from build123d import *

# Parameters (mm, degrees)
F2_W        = 15
F2_H        = 19.25
F2_R        = 2.75
F3_DEPTH    = 40
F5_DEPTH    = 22.251
F6_W        = 6.75
F6_H        = 19.25
F6_W_2      = 20.5
F7_DEPTH    = 30.001
F8_T1_DEPTH = 15
F8_T3_DEPTH = 28
F8_T5_DEPTH = 28
F8_T7_DEPTH = 28
F10_R       = 2


# Not quite as in the source:
# - a fillet or chamfer that OpenCascade refuses, or shapes differently, is made with other operations: its cross-section is extruded or revolved along the edge and cut away or added
# - a feature of the source that left no trace in its solid (it failed there, or was rolled back) is left out


with BuildPart() as f3:
    # F2 (on Front) → F3 (new body)
    with BuildSketch(Plane.XZ):
        Polygon((-47, -12.4571), (-32, -12.4571), (-17, -12.4571), (-17, -9.4571), (-47, -9.4571), align=None)
        with Locations((-39.5, -22.0821)):
            Rectangle(F2_W, F2_H)
        with Locations((-39.5, -23.9571)):
            Circle(F2_R, mode=Mode.SUBTRACT)
    extrude(amount=F3_DEPTH)

    # F4 (on face) → F5 (cut, through all)
    with BuildSketch(Plane.XY.offset(-9.4571)):
        with BuildLine():
            Line((-24, -11.5), (-24, -6.5))
            ThreePointArc((-24, -6.5), (-26, -4.5), (-28, -6.5))
            Line((-28, -6.5), (-28, -11.5))
            ThreePointArc((-28, -11.5), (-26, -13.5), (-24, -11.5))
        make_face()
        with BuildLine():
            Line((-32, -22.5), (-32, -17.5))
            ThreePointArc((-32, -17.5), (-34, -15.5), (-36, -17.5))
            Line((-36, -17.5), (-36, -22.5))
            ThreePointArc((-36, -22.5), (-34, -24.5), (-32, -22.5))
        make_face()
        with BuildLine():
            ThreePointArc((-28, -33.5), (-26, -35.5), (-24, -33.5))
            Line((-24, -33.5), (-24, -28.5))
            ThreePointArc((-24, -28.5), (-26, -26.5), (-28, -28.5))
            Line((-28, -28.5), (-28, -33.5))
        make_face()
    extrude(amount=-F5_DEPTH, mode=Mode.SUBTRACT)

    # F6 (on face) → F7 (cut, through all)
    with BuildSketch(Plane(origin=(-47, 0, 0), x_dir=(0, -1, 0), z_dir=(-1, 0, 0))):
        with Locations((3.375, -22.0821)):
            Rectangle(F6_W, F6_H)
        with Locations((20, -22.0821)):
            Rectangle(F6_W_2, F6_H)
        with Locations((36.625, -22.0821)):
            Rectangle(F6_W, F6_H)
    extrude(amount=-F7_DEPTH, mode=Mode.SUBTRACT)

    # F8: fillet of radius 5 on 10 edges, made by hand

    # F8_s2 → F8_t1 (join)
    with BuildSketch(Plane.YZ.offset(-47)):
        with BuildLine():
            ThreePointArc((-1.75, -12.4571), (-5.2855339059, -13.9215660941), (-6.75, -17.4571))
            Line((-6.75, -17.4571), (-6.75, -12.4571))
            Line((-6.75, -12.4571), (-1.75, -12.4571))
        make_face()
        with BuildLine():
            ThreePointArc((-38.25, -12.4571), (-34.7144660941, -13.9215660941), (-33.25, -17.4571))
            Line((-33.25, -17.4571), (-33.25, -12.4571))
            Line((-33.25, -12.4571), (-38.25, -12.4571))
        make_face()
    extrude(amount=F8_T1_DEPTH)

    # F8_s4 → F8_t3 (cut)
    with BuildSketch(Plane.XY.offset(-24.9571)):
        with BuildLine():
            ThreePointArc((-17, -5), (-18.4644660941, -1.4644660941), (-22, 0))
            Line((-22, 0), (-17, 0))
            Line((-17, 0), (-17, -5))
        make_face()
        with BuildLine():
            ThreePointArc((-17, -35), (-18.4644660941, -38.5355339059), (-22, -40))
            Line((-22, -40), (-17, -40))
            Line((-17, -40), (-17, -35))
        make_face()
        with BuildLine():
            ThreePointArc((-47, -5), (-45.5355339059, -1.4644660941), (-42, 0))
            Line((-42, 0), (-47, 0))
            Line((-47, 0), (-47, -5))
        make_face()
        with BuildLine():
            ThreePointArc((-42, -40), (-45.5355339059, -38.5355339059), (-47, -35))
            Line((-47, -35), (-47, -40))
            Line((-47, -40), (-42, -40))
        make_face()
    extrude(amount=F8_T3_DEPTH, mode=Mode.SUBTRACT)

    # F8_s6 → F8_t5 (cut)
    with BuildSketch(Plane.XZ.offset(17.75)):
        with BuildLine():
            ThreePointArc((-42, -31.7071), (-45.5355339059, -30.2426339059), (-47, -26.7071))
            Line((-47, -26.7071), (-47, -31.7071))
            Line((-47, -31.7071), (-42, -31.7071))
        make_face()
        with BuildLine():
            ThreePointArc((-37, -31.7071), (-33.4644660941, -30.2426339059), (-32, -26.7071))
            Line((-32, -26.7071), (-32, -31.7071))
            Line((-32, -31.7071), (-37, -31.7071))
        make_face()
    extrude(amount=F8_T5_DEPTH, mode=Mode.SUBTRACT)

    # F8_s8 → F8_t7 (cut)
    with BuildSketch(Plane.XZ.offset(-5.75)):
        with BuildLine():
            ThreePointArc((-42, -31.7071), (-45.5355339059, -30.2426339059), (-47, -26.7071))
            Line((-47, -26.7071), (-47, -31.7071))
            Line((-47, -31.7071), (-42, -31.7071))
        make_face()
        with BuildLine():
            ThreePointArc((-37, -31.7071), (-33.4644660941, -30.2426339059), (-32, -26.7071))
            Line((-32, -26.7071), (-32, -31.7071))
            Line((-32, -31.7071), (-37, -31.7071))
        make_face()
    extrude(amount=F8_T7_DEPTH, mode=Mode.SUBTRACT)

    # F10
    f10_edges = [f3.edges().sort_by_distance(p)[0] for p in [
        (-39.5, -30.25, -12.4571),
        (-39.5, -9.75, -12.4571),
        (-32, -34.25, -12.4571),
        (-32, -5.75, -12.4571),
    ]]
    fillet(f10_edges, radius=F10_R)


solid = f3.part
Part model, mm, in its own coordinate system. A direction names the side the tool comes from. Coordinates: 2 decimals unless noted, no trailing zeros. Order: outer loops, then holes, each group sorted by start corner. A loop starts at its lowest first (then second) coordinate and runs counter-clockwise, first axis right, second up. Notation, with made-up numbers: M 35.25,-17 L 89.25,-17 A27 cw 89.25,4 Z; hole C 2.25,65 d4. An arc over 180 degrees is marked long. Use a Markdown table: item, result.
(1) Flat gauge pins, fed straight in: pin 1 (2 mm diameter, centred on y = -7, z = -22, fed in from +X); pin 2 (4.5 mm diameter, centred on x = -43, z = -26, fed in from -Y); pin 3 (1.5 mm diameter, centred on x = -30, z = -21.5, fed in from -Y); pin 4 (6.5 mm diameter, centred on x = -39.5, z = -23.96, fed in from +Y). Where does each tip first touch, or does it go through?
A:
| item | result |
|---|---|
| pin 1 | stops at x = -32 |
| pin 2 | stops at y = -33.25 |
| pin 3 | passes through |
| pin 4 | stops at y = -6.75 |
(2) Cut at B-B on y = -19. Write the cut outline in (x, z), then the cut area to 3 significant figures.
A:
| item | result |
|---|---|
| outline | M -47,-12.46 L -36,-12.46 L -36,-9.46 L -47,-9.46 Z; M -32,-12.46 L -17,-12.46 L -17,-9.46 L -32,-9.46 Z |
| area | 78.0 mm^2 |
(3) Cut at D-D on x = -33. Write the cut outline in (y, z), then the cut area to 3 significant figures.
A:
| item | result |
|---|---|
| outline | M -40,-12.46 L -38.25,-12.46 A5 cw -33.25,-17.46 L -33.25,-29.71 L -30.25,-29.71 L -30.25,-14.46 A2 cw -28.25,-12.46 L -24.23,-12.46 L -24.23,-9.46 L -40,-9.46 Z; M -15.77,-12.46 L -11.75,-12.46 A2 cw -9.75,-14.46 L -9.75,-29.71 L -6.75,-29.71 L -6.75,-17.46 A5 cw -1.75,-12.46 L 0,-12.46 L 0,-9.46 L -15.77,-9.46 Z |
| area | 211 mm^2 |
(4) Pull direction Y, two halves, no side cores. Call faces 1 (the flat face through (-31.8, -19.7, -9.457)), 2 (the flat face through (-24, -31, -11)), 3 (the cylindrical face through (-38.619, -5.246, -13.883)): released by +Y, released by -Y, zero draft, split by the parting line, or undercut.
A:
| item | result |
|---|---|
| face 1 | zero draft |
| face 2 | undercut |
| face 3 | released by +Y |
(5) Cut at C-C on x = -26. Write the cut outline in (y, z), then the cut area to 3 significant figures.
A:
| item | result |
|---|---|
| outline | M -40,-12.46 L -35.5,-12.46 L -35.5,-9.46 L -40,-9.46 Z; M -26.5,-12.46 L -13.5,-12.46 L -13.5,-9.46 L -26.5,-9.46 Z; M -4.5,-12.46 L 0,-12.46 L 0,-9.46 L -4.5,-9.46 Z |
| area | 66.0 mm^2 |
(6) Cut at A-A on z = -19.5. Write the cut outline in (x, y).
A:
| item | result |
|---|---|
| outline | M -47,-33.25 L -32,-33.25 L -32,-30.25 L -47,-30.25 Z; M -47,-9.75 L -32,-9.75 L -32,-6.75 L -47,-6.75 Z |
(7) Probe L1, parallel to Y at x = -33, z = -28.75; L2, parallel to Z at x = -39.5, y = -8. List the from-to ranges inside material, lowest first.
A:
| item | result |
|---|---|
| L1 | y = -33.25 to -30.25, -9.75 to -6.75 |
| L2 | z = -31.71 to -26.71, -21.21 to -9.46 |
(8) Tool access for faces 4 (the flat face through (-41, -9.75, -21)), 5 (the cylindrical face through (-34, -24.5, -10.9)), 6 (the cylindrical face through (-41.682, -8.229, -25.63)): list every direction of +Z, -Z, +X, -X, +Y, -Y with a clear straight run to the whole face (end or side of a thin tool).
A:
| item | result |
|---|---|
| face 4 | -Z, +X, -X |
| face 5 | +Z, -Z |
| face 6 | +Y, -Y |
